CAD build for the part. Positions are in the model's coordinates, mm. A direction names the side the tool comes from. Give positions to 0.01 mm unless a question says otherwise; leave off trailing zeros. Write each loop counter-clockwise with the first axis right and the second up, starting at its lowest first coordinate (ties: lowest second). Pieces come first, ordered by that corner, then holes. Notation, with made-up numbers: (24, 40) -> (37, 40) arc R13 cw to (37, 57) -> close; hole circle Ø6 at (-18, -14). An arc over 180 degrees is marked (long way). Answer as a JSON object with one key per item and string values.
```python
from build123d import *

# Parameters (mm, degrees)
SKETCH011_AS_DRAWN_W                 = 10
SKETCH011_AS_DRAWN_H                 = 3
EXTRUDE005_DEPTH                     = 10
EXTRUDE005_ONTO_SKETCH011_ROLL_ANGLE = 90
BOX_W                                = 11
BOX_H                                = 11
BOX_DEPTH                            = 10
FILLET001_R                          = 1
SKETCH007_W                          = 62.8586
SKETCH007_H                          = 35
EXTRUDE003_DEPTH                     = 5
CYLINDER_R                           = 2
CYLINDER_DEPTH                       = 40
SKETCH003_W                          = 44
SKETCH003_H                          = 77
PAD_DEPTH                            = 30
THICKNESS_T                          = 1.5
SKETCH005_R                          = 2
SKETCH005_R_2                        = 1
PAD001_DEPTH                         = 3
EXTRUDE004_DEPTH                     = 5


with BuildPart() as extrude005:
    # Sketch011 as drawn → Extrude005 (new)
    with BuildSketch(Plane.XY):
        with Locations((10.197845, 12.338122)):
            Rectangle(SKETCH011_AS_DRAWN_W, SKETCH011_AS_DRAWN_H)
    extrude(amount=-EXTRUDE005_DEPTH)


with BuildPart() as extrude005_1:
    # Extrude005 onto Sketch011 roll: moved
    add(extrude005.part.rotate(Axis((0, 0, 0), (1, 0, 0)), EXTRUDE005_ONTO_SKETCH011_ROLL_ANGLE))


with BuildPart() as extrude005_2:
    # Extrude005 onto Sketch011 placement: moved
    add(extrude005_1.part.moved(Location((0, -139, 0))))


with BuildPart() as fillet001:
    # Box → Box (new body)
    with BuildSketch(Plane.XY):
        with Locations((5.5, 5.5)):
            Rectangle(BOX_W, BOX_H)
    extrude(amount=BOX_DEPTH)

    # Fillet001
    fillet001_edges = [fillet001.edges().sort_by_distance(p)[0] for p in [
        (0, 0, 5),
        (0, 11, 5),
        (11, 0, 5),
        (11, 11, 5),
    ]]
    fillet(fillet001_edges, radius=FILLET001_R)


with BuildPart() as fillet001_1:
    # Fillet001 placement: moved
    add(fillet001.part.moved(Location((-1, -118, 14))))


with BuildPart() as extrude003:
    # Sketch007 → Extrude003 (new body)
    with BuildSketch(Plane.XY):
        with Locations((11.4293, -93.929395)):
            Rectangle(SKETCH007_W, SKETCH007_H)
    extrude(amount=EXTRUDE003_DEPTH)


with BuildPart() as cilindro:
    # Cylinder → Cylinder (new body)
    with BuildSketch(Plane(origin=(-29, 21, -2), x_dir=(1, 0, 0), z_dir=(0, 0, 1))):
        Circle(CYLINDER_R)
    extrude(amount=CYLINDER_DEPTH)


with BuildPart() as cut:
    # Sketch003 → Pad (new body)
    with BuildSketch(Plane(origin=(0, 0, 0), x_dir=(-1, 0, 0), z_dir=(0, 0, -1))):
        with Locations((22, 38.5)):
            Rectangle(SKETCH003_W, SKETCH003_H)
    extrude(amount=PAD_DEPTH)

    # Thickness
    thickness_openings = [cut.faces().sort_by_distance(p)[0] for p in [
        (-22, 38.5, -30),
    ]]
    offset(amount=THICKNESS_T, openings=thickness_openings)


with BuildPart() as cut_1:
    # Thickness placement: moved
    add(cut.part.moved(Location((9e-06, 2.6e-05, 20.905646))))

    # Cut: cut Cilindro
    add(cilindro.part, mode=Mode.SUBTRACT)


with BuildPart() as cut003:
    # Sketch005 → Pad001 (new body)
    with BuildSketch(Plane(origin=(0, 0, 21), x_dir=(1, 0, 0), z_dir=(0, 0, -1))):
        with Locations((-32, -10)):
            Circle(SKETCH005_R)
        with Locations((-32, -10)):
            Circle(SKETCH005_R_2, mode=Mode.SUBTRACT)
    extrude(amount=PAD001_DEPTH)

    # Fusion: union Cut
    add(cut_1.part)


with BuildPart() as cut003_1:
    # Fusion placement: moved
    add(cut003.part.moved(Location((32.999991, -134.000034, 9.094354))))

    # Cut001: cut Extrude003
    add(extrude003.part, mode=Mode.SUBTRACT)


with BuildPart() as cut003_2:
    # Cut001 placement: moved
    add(cut003_1.part.moved(Location((0, 0, -9.094209))))

    # Cut002: cut Fillet001
    add(fillet001_1.part, mode=Mode.SUBTRACT)

    # Cut003: cut Extrude005
    add(extrude005_2.part, mode=Mode.SUBTRACT)


with BuildPart() as fusion002:
    # Sketch009 → Extrude004 (new body)
    with BuildSketch(Plane.YZ.offset(15)):
        Polygon((-79.324959, 21), (-79.324959, 15), (-82.324959, 15), (-82.324959, 16), (-81.324959, 16), (-81.324959, 18), (-83.324959, 18), (-83.324959, 21), align=None)
    extrude(amount=EXTRUDE004_DEPTH)

    # Fusion002: union Cut003
    add(cut003_2.part)


solid = fusion002.part
```
1) Pin check, flat tips, straight feed: pin 1 (4 mm diameter, centred on x = 6.5, y = -81, fed in from -Z); pin 2 (22 mm diameter, centred on x = 19.5, y = -82.5, fed in from -Z); pin 3 (3 mm diameter, centred on x = 0.5, y = -123, fed in from -Z); pin 4 (1.6 mm diameter, centred on y = -134.5, z = 13, fed in from -X). Stop position of each tip, or through.
Model answer:
{"pin 1": "stops at z = 20.91", "pin 2": "stops at z = 15", "pin 3": "stops at z = 18", "pin 4": "stops at x = -12.5"}
2) Slice it at A-A (x = 8). List the corners of the cut face in (y, z).
Model answer:
{"outline": "(-135.5, -9.09) -> (-134, -9.09) -> (-134, 10.84) -> (-135.5, 10.84) -> close; (-135.5, 13.84) -> (-134, 13.84) -> (-134, 20.91) -> (-118, 20.91) -> (-118, 22.41) -> (-134, 22.41) arc R1.5 ccw to (-135.5, 20.91) -> close; (-107, 20.91) -> (-57, 20.91) -> (-57, -9.09) -> (-55.5, -9.09) -> (-55.5, 20.91) arc R1.5 ccw to (-57, 22.41) -> (-107, 22.41) -> close"}
3) Slice it at C-C (z = 6). List the corners of the cut face in (x, y).
Model answer:
{"outline": "(-12.5, -134) arc R1.5 ccw to (-11, -135.5) -> (33, -135.5) arc R1.5 ccw to (34.5, -134) -> (34.5, -57) arc R1.5 ccw to (33, -55.5) -> (-11, -55.5) arc R1.5 ccw to (-12.5, -57) -> close; hole (-11, -134) -> (33, -134) -> (33, -57) -> (-11, -57) -> close"}
4) 3-axis set-ups, long thin cutter, end or side, ignore diameter. For faces 1 (the flat face through (1, -124, 20.906)), 2 (the flat face through (34, -111.429, -7)), 3 (the flat face through (10, -135, 13.838)), 4 (the flat face through (-1, -113, 22)): which of +Z, -Z, +X, -X, +Y, -Y reach the whole face in a straight line?
Model answer:
{"face 1": "-Z", "face 2": "-Z, +X, -X", "face 3": "-Y", "face 4": "+Z, -Z"}
5) Slice it at D-D (z = 20). List the corners of the cut face in (x, y).
Model answer:
{"outline": "(-12.5, -134) arc R1.5 ccw to (-11, -135.5) -> (33, -135.5) arc R1.5 ccw to (34.5, -134) -> (34.5, -57) arc R1.5 ccw to (33, -55.5) -> (-11, -55.5) arc R1.5 ccw to (-12.5, -57) -> close; circle Ø4 at (1, -124); (15, -83.32) -> (20, -83.32) -> (20, -79.32) -> (15, -79.32) -> close; hole (-11, -134) -> (33, -134) -> (33, -57) -> (-11, -57) -> close; hole circle Ø2 at (1, -124)"}
6) Wall check: probe 1 along Y at (x, z) = (14.5, 17); probe 2 along X at (y, z) = (-79, 20.5); probe 3 along Y at (x, z) = (5, 21). Give the ranges that are in metal, low to high.
Model answer:
{"probe 1": "y = -135.5 to -134, -57 to -55.5", "probe 2": "x = -12.5 to -11, 33 to 34.5", "probe 3": "y = -135.5 to -118, -107 to -55.5"}
7) Mould opens along Y. For faces 5 (the flat face through (2, -123, 18)), 6 (the cylindrical face through (-12.072, -94.961, 21.955)), 7 (the cylindrical face through (-12.07, -55.95, 5.7)) say: released by +Y, released by -Y, zero draft, split by the parting line, or undercut.
Model answer:
{"face 5": "undercut", "face 6": "zero draft", "face 7": "released by +Y"}
8) Slice it at B-B (y = -72). List the corners of the cut face in (x, z).
Model answer:
{"outline": "(-12.5, -9.09) -> (-11, -9.09) -> (-11, 20.91) -> (33, 20.91) -> (33, -9.09) -> (34.5, -9.09) -> (34.5, 20.91) arc R1.5 ccw to (33, 22.41) -> (-11, 22.41) arc R1.5 ccw to (-12.5, 20.91) -> close"}
